Geometry: final body of the model. Coordinates: model frame, mm. Face numbers are marked on the shaded views. Coordinates: 2 decimals unless noted, no trailing zeros. Loops run counter-clockwise (first coordinate to the right, second up) from the corner with the lowest first, then second, coordinate; pieces in that order, holes last. Notation, with made-up numbers: (76, 62) - (114, 62) arc R20 cw to (114, 86) - close; hole circle Ø6 at (-29.5, 63). An arc over 180 degrees is marked (long way). Write each question's results on one line, items separated by ' | '. Start each with the question number.
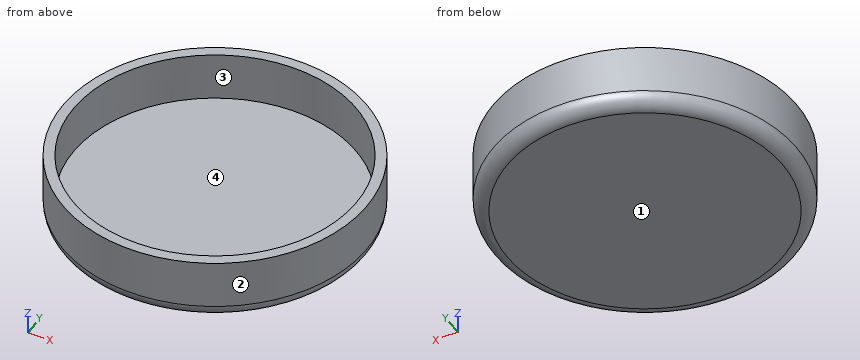
from build123d import *

# Parameters (mm, degrees)
F0_R     = 21.75
F1_DEPTH = 2
F2_R     = 21.75
F2_R_2   = 20.25
F3_DEPTH = 9
F4_R     = 2


with BuildPart() as f1:
    # F0 (on Top) → F1 (new body)
    with BuildSketch(Plane.XY):
        Circle(F0_R)
    extrude(amount=F1_DEPTH)

    # F2 (on Top) → F3 (join)
    with BuildSketch(Plane.XY):
        Circle(F2_R)
        Circle(F2_R_2, mode=Mode.SUBTRACT)
    extrude(amount=F3_DEPTH)

    # F4
    f4_edges = [f1.edges().sort_by_distance(p)[0] for p in [
        (-21.75, 0, 0),
    ]]
    fillet(f4_edges, radius=F4_R)


solid = f1.part
1) Section query A-A on z = 4.25. Output: boundary loops of the cut face in (x, y), and give its area (3 significant figures).
2) Section query B-B on x = 0. Output: boundary loops of the cut face in (y, z), and give its area (3 significant figures).
3) Material intervals for line 1 (Y direction, x = 0, z = 6.75); line 2 (Z direction, x = -1.5, y = 8.5); line 3 (X direction, y = -17, z = 8.5), sorted ascending. Write a range as [from, to].
4) Pin query (flat end, axial travel): pin 1 Ø10 at (x, y) = (11.5, -5) entering from +Z. Return the tip coordinate at first contact, or that it passes through.
5) Pull-direction query (Y, two-part tool) for the marked faces 1, 2, 3 and 4; classes: released by +Y, released by -Y, zero draft, split by the parting line, or undercut.
Returned:
1) outline: circle Ø43.5 at (0, 0); hole circle Ø40.5 at (0, 0) | area: 198 mm²
2) outline: (-21.75, 2) arc R2 ccw to (-19.75, 0) - (19.75, 0) arc R2 ccw to (21.75, 2) - (21.75, 9) - (20.25, 9) - (20.25, 2) - (-20.25, 2) - (-20.25, 9) - (-21.75, 9) - close | area: 106 mm²
3) line 1: y = [-21.75, -20.25], [20.25, 21.75] | line 2: z = [0, 2] | line 3: x = [-13.57, -11], [11, 13.57]
4) pin 1: stops at z = 2
5) face 1: zero draft | face 2: split by the parting line | face 3: undercut | face 4: undercut
